Verification items for the finished model (mm, model axes). A direction names the side the tool comes from. Round coordinates to 2 decimals unless told otherwise and drop trailing zeros. Write each loop counter-clockwise with the first axis right and the second up, starting at its lowest first coordinate (ties: lowest second). Pieces come first, ordered by that corner, then holes. Notation, with made-up numbers: M 36,26.25 L 73,26.25 A17 ccw 73,47.25 Z; hole C 70.5,-32.75 d5. An arc over 180 degrees is marked long. Answer in a Markdown table with one row per item. Add a question column.
1. Go/stop test with flat-tipped pins: pin 1 Ø1 at (x, y) = (1.5, 0) entering from -Z; pin 2 Ø2 at (y, z) = (2, 0) entering from +X; pin 3 Ø0.7 at (y, z) = (-0.5, 1) entering from +X (3 decimals). Record where each tip stops, or that it passes through.
2. Set-up check for faces 1 (the flat face through (-1, -1, 0)), 2 (the cylindrical face through (-0.488, -2.196, 0.558)): record each of +Z, -Z, +X, -X, +Y, -Y from which the full face is reachable in a straight line by a thin tool's end or side.
3. Sectioned sample at B-B on z = -3.2. Record the cut outline in (x, y), plus the area to 3 significant figures.
4. Sectioned sample at A-A on y = 0. Record the cut outline in (x, z).
5. Sectioned sample at D-D on z = 0.25. Record the cut outline in (x, y).
6. Sectioned sample at C-C on x = -0.2. Record the cut outline in (y, z), plus the area to 3 significant figures.
7. Material ranges on probe 1 along X at (y, z) = (-0.1, 1.3); probe 2 along Z at (x, y) = (1.1, 1.2); probe 3 along Y at (x, z) = (-1, -1.9), recorded low to high.
```python
from build123d import *

# Parameters (mm, degrees)
F2_W          = 0.6
F2_H          = 0.6
F3_DEPTH      = 2.251
F3_DEPTH_BACK = 2.251


with BuildPart() as f1:
    # F0 (on Front) → F1 (revolve)
    with BuildSketch(Plane.XZ):
        with BuildLine():
            Line((1.75, 1.6), (0, 1.6))
            Line((0, 1.6), (0, -4))
            Line((0, -4), (1.25, -4))
            Line((1.25, -4), (1.25, 0))
            Line((1.25, 0), (2.25, 0))
            Line((2.25, 0), (2.25, 1.1))
            ThreePointArc((2.25, 1.1), (2.1035533906, 1.4535533906), (1.75, 1.6))
        make_face()
    revolve(axis=Axis((0, 0, 1.6484611327), (0, 0, 1)))

    # F2 (on Front) → F3 (cut, two sides)
    with BuildSketch(Plane.XZ) as f3_sk:
        with Locations((0, 1.3)):
            Rectangle(F2_W, F2_H)
    extrude(amount=-F3_DEPTH, mode=Mode.SUBTRACT)
    extrude(f3_sk.sketch, amount=F3_DEPTH_BACK, mode=Mode.SUBTRACT)


solid = f1.part
```
Geometry check:
| question | item | result |
|---|---|---|
| 1 | pin 1 | stops at z = -4 |
| 1 | pin 2 | stops at x = 2.02 |
| 1 | pin 3 | stops at x = 2.245 |
| 2 | face 1 | -Z |
| 2 | face 2 | +Z, -Z |
| 3 | outline | C 0,0 d2.5 |
| 3 | area | 4.91 mm2 |
| 4 | outline | M -2.25,0 L -1.25,0 L -1.25,-4 L 1.25,-4 L 1.25,0 L 2.25,0 L 2.25,1.1 A0.5 ccw 1.75,1.6 L 0.3,1.6 L 0.3,1 L -0.3,1 L -0.3,1.6 L -1.75,1.6 A0.5 ccw -2.25,1.1 Z |
| 5 | outline | C 0,0 d4.5 |
| 6 | outline | M -2.24,0 L -1.23,0 L -1.23,-4 L 1.23,-4 L 1.23,0 L 2.24,0 L 2.24,1 L -2.24,1 Z |
| 6 | area | 14.4 mm2 |
| 7 | probe 1 | x = -2.21 to -0.3, 0.3 to 2.21 |
| 7 | probe 2 | z = 0 to 1.6 |
| 7 | probe 3 | y = -0.75 to 0.75 |
